from build123d import *

# Parameters (mm, degrees)
F0_R          = 18
F0_R_2        = 13.5
F1_DEPTH      = 4
F0_R_3        = 12
F2_DEPTH      = 0.5
F2_DEPTH_BACK = 0.1
F3_SIZE       = 1
F4_SIZE       = 1


with BuildPart() as f1:
    # F0 (on Top) → F1 (new body)
    with BuildSketch(Plane.XY):
        Circle(F0_R)
        Circle(F0_R_2, mode=Mode.SUBTRACT)
    extrude(amount=F1_DEPTH)

    # F0 (on Top) → F2 (join, two sides)
    with BuildSketch(Plane.XY) as f2_sk:
        Circle(F0_R_2)
        Circle(F0_R_3, mode=Mode.SUBTRACT)
    extrude(amount=-F2_DEPTH)
    extrude(f2_sk.sketch, amount=F2_DEPTH_BACK)

    # F3
    f3_edges = [f1.edges().sort_by_distance(p)[0] for p in [
        (-13.5, 0, 0.1),
    ]]
    chamfer(f3_edges, length=F3_SIZE)

    # F4
    f4_edges = [f1.edges().sort_by_distance(p)[0] for p in [
        (-18, 0, 4),
        (-13.5, 0, 4),
    ]]
    chamfer(f4_edges, length=F4_SIZE)


solid = f1.part
Geometry: final body of the model. Coordinates: model frame, mm. A direction names the side the tool comes from. Round coordinates to 2 decimals unless told otherwise and drop trailing zeros. Order: outer loops, then holes, each group sorted by start corner. A loop starts at its lowest first (then second) coordinate and runs counter-clockwise, first axis right, second up.
Q1. Section A-A, the plane y = 0. Output: boundary loops of the cut face in (x, z).
Result sheet:
outline: (-18, 0) - (-13.5, 0) - (-13.5, -0.5) - (-12, -0.5) - (-12, 0.1) - (-12.5, 0.1) - (-13.5, 1.1) - (-13.5, 3) - (-14.5, 4) - (-17, 4) - (-18, 3) - close; (12, -0.5) - (13.5, -0.5) - (13.5, 0) - (18, 0) - (18, 3) - (17, 4) - (14.5, 4) - (13.5, 3) - (13.5, 1.1) - (12.5, 0.1) - (12, 0.1) - close
Q2. Material intervals for probe 1 along Y at (x, z) = (0, -0.25); probe 2 along Y at (x, z) = (0, 2.05); probe 3 along X at (y, z) = (3.5, 1.35), sorted ascending.
Result sheet:
probe 1: y = -13.5 to -12, 12 to 13.5
probe 2: y = -18 to -13.5, 13.5 to 18
probe 3: x = -17.66 to -13.04, 13.04 to 17.66
Q3. Mould query, pull axis X, two halves, no side actions, for faces 1 (the face through (-2.93, -13.18, -0.25)), 2 (the face through (-11.99, 0.53, -0.2)), 3 (the face through (2.58, 13.42, 0)), 4 (the face through (-2.93, -13.18, 2.04)). Classes: released by +X, released by -X, zero draft, split by the parting line, or undercut.
Result sheet:
face 1: split by the parting line
face 2: undercut
face 3: zero draft
face 4: undercut
Q4. Access query for faces 5 (the face through (-2.343, 17.847, 1.479)), 6 (the face through (-7, 10, 0.1)). Directions: +Z, -Z, +X, -X, +Y, -Y. A direction counts if a zero-diameter tool reaches every point of the face in a straight line with its end or side. Return the directions, or none.
Result sheet:
face 5: +Z, -Z
face 6: +Z
